Build history of the part. All positions in model axes, mm. Give positions to 0.01 mm unless a question says otherwise; leave off trailing zeros. Loops run counter-clockwise (first coordinate to the right, second up) from the corner with the lowest first, then second, coordinate; pieces in that order, holes last. Notation, with made-up numbers: (-7, 40) -> (34, 40) arc R12 ccw to (34, 50) -> close; hole circle Ø11 at (44.5, 58.25). An arc over 180 degrees is marked (long way). Answer in a Markdown table with one row per item. Add a question column.
from build123d import *

# Parameters (mm, degrees)
MAIN_SHAPE_PROFILE_W    = 28.575
MAIN_SHAPE_PROFILE_H    = 6.35
DOWEL_HOLES_PROFILE_R   = 1.27
DOWEL_HOLES_DEPTH       = 2.54
F_3_8_16_TAPPED_HOLE1_D = 1.2954


with BuildPart() as part:
    # Main Shape Profile → Main Shape (revolve)
    with BuildSketch(Plane.XY, mode=Mode.PRIVATE) as main_shape_sk:
        with Locations((14.2875, 3.175)):
            Rectangle(MAIN_SHAPE_PROFILE_W, MAIN_SHAPE_PROFILE_H)
    revolve(main_shape_sk.sketch.rotate(Axis((0, 0, 0), (0, -1, 0)), 90), axis=Axis((0, 0, 0), (0, -1, 0)))

    # Dowel Holes Profile → Dowel Holes (cut)
    with BuildSketch(Plane.XZ):
        with Locations(Location((0, 25.4, 0), (0, 0, 270))):
            Circle(DOWEL_HOLES_PROFILE_R)
        with Locations(Location((0, -25.4, 0), (0, 0, 270))):
            Circle(DOWEL_HOLES_PROFILE_R)
    extrude(amount=-DOWEL_HOLES_DEPTH, mode=Mode.SUBTRACT)

    # 3/8-16 Tapped Hole1 (through all)
    with Locations(Plane(origin=(0, 6.35, 0), x_dir=(1, 0, 0), z_dir=(0, 1, 0))):
        with Locations((-5.971898163, -8.219612663), (0, -13.97), (0, -17.78), (-9.662734206, -3.139612663), (-9.662734206, 3.139612663), (-5.971898163, 8.219612663), (0, 10.16), (5.971898163, 8.219612663), (9.662734206, 3.139612663), (9.662734206, -3.139612663), (5.971898163, -8.219612663), (0, -10.16), (-6.061355835, -12.586535085), (-10.92218581, -8.710152532), (-13.619742933, -3.108617447), (-13.619742933, 3.108617447), (-10.92218581, 8.710152532), (-6.061355835, 12.586535085), (0, 13.97), (6.061355835, 12.586535085), (10.92218581, 8.710152532), (13.619742933, 3.108617447), (13.619742933, -3.108617447), (10.92218581, -8.710152532), (6.061355835, -12.586535085), (-6.081118148, -16.707734798), (-11.4287637, -13.620270199), (-15.397931679, -8.89), (-17.509881849, -3.087464599), (-17.509881849, 3.087464599), (-15.397931679, 8.89), (-11.4287637, 13.620270199), (-6.081118148, 16.707734798), (0, 17.78), (6.081118148, 16.707734798), (11.4287637, 13.620270199), (15.397931679, 8.89), (17.509881849, 3.087464599), (17.509881849, -3.087464599), (15.397931679, -8.89), (11.4287637, -13.620270199), (6.081118148, -16.707734798)):
            Hole(F_3_8_16_TAPPED_HOLE1_D / 2)


solid = part.part
(1) Saw through at C-C, the plane x = 24.5. List the corners of the cut face in (y, z).
(2) Saw through at A-A, the plane z = -25.4. List the corners of the cut face in (x, y).
(3) Two-plate mould, pull along X, no slides. Class faces 1 (the flat face through (0, 0, 0)), 2 (the cylindrical face through (-16.016, 3.131, 8.695)), 3 (the cylindrical face through (-6.679, 3.131, 16.956)): released by +X, released by -X, zero draft, split by the parting line, or undercut.
(4) Saw through at D-D, the plane z = 6. List the corners of the cut face in (x, y), then the cut area to 3 significant figures.
(5) Saw through at B-B, the plane y = 1.75. State how many separate pieces and enclosed holes the cut face has, then the cut area to 3 significant figures.
(6) Flat gauge pins, fed straight in: pin 1 Ø3 at (x, y) = (-5, 2.5) entering from +Z; pin 2 Ø2 at (x, z) = (0, -25.4) entering from -Y; pin 3 Ø2 at (y, z) = (1, -12) entering from +X. Where does each tip first touch, or does it go through?
(7) Wall check: line 1 along Z through (x, y) = (10.5, 2.5); line 2 along X through (y, z) = (3.75, -8); line 3 along Z through (x, y) = (-12, 1.25). Give the ranges that are in metal, low to high. Write a range as from..to.
Worked answers:
| question | item | result |
|---|---|---|
| 1 | outline | (0, -14.71) -> (6.35, -14.71) -> (6.35, 14.71) -> (0, 14.71) -> close |
| 2 | outline | (-13.09, 0) -> (-1.27, 0) -> (-1.27, 2.54) -> (1.27, 2.54) -> (1.27, 0) -> (13.09, 0) -> (13.09, 6.35) -> (-13.09, 6.35) -> close |
| 3 | face 1 | zero draft |
| 3 | face 2 | undercut |
| 3 | face 3 | undercut |
| 4 | outline | (-27.94, 0) -> (27.94, 0) -> (27.94, 6.35) -> (-27.94, 6.35) -> close |
| 4 | area | 355 mm^2 |
| 5 | separate pieces | 1 |
| 5 | enclosed holes | 44 |
| 5 | area | 2,500 mm^2 |
| 6 | pin 1 | z = 28.36 |
| 6 | pin 2 | y = 2.54 |
| 6 | pin 3 | x = 26.37 |
| 7 | line 1 | -26.58..-9.2, -8.22..8.22, 9.2..26.58 |
| 7 | line 2 | -27.43..-6.58, -5.36..5.36, 6.58..27.43 |
| 7 | line 3 | -25.93..-13.93, -13.31..13.31, 13.93..25.93 |
